Geometry check sheet. Reference: the model listing, model coordinates, mm. A direction names the side the tool comes from. Coordinates: 2 decimals unless noted, no trailing zeros. Write each loop counter-clockwise with the first axis right and the second up, starting at its lowest first coordinate (ties: lowest second). Pieces come first, ordered by that corner, then holes. Notation, with made-up numbers: (-9, -2) -> (-4, -2) arc R22 ccw to (-4, 7) -> close; hole circle Ø3 at (1, 53). An arc over 180 degrees is marked (long way). Use a Markdown table: item, result.
Autodesk Inventor part; units mm, degrees
ref_plane "Pracovní rovina2" through (15, 0, 0) normal (1, 0, 0) x (0, 0, -1)
ref_plane "YZ Plane" through (0, 0, 0) normal (1, 0, 0) x (0, 1, 0)
ref_plane "XZ Plane" through (0, 0, 0) normal (0, 1, 0) x (-1, 0, 0)
sketch "Náčrt1" plane through (0, 0, 0) normal (1, 0, 0) x (0, 1, 0)
  line L0 (0, 0) -> (100, 0)
  line L1 (100, 0) -> (100, -6)
  line L2 (100, -6) -> (6, -6)
  line L3 (6, -6) -> (6, -100)
  line L4 (6, -100) -> (0, -100)
  line L5 (0, -100) -> (0, 0)
  point P0 (100, -148)
  point P1 (100, -150)
  dimension "d0" = 100
  dimension "d1" = 6
  dimension "d20" = 100
  dimension "d40" = 6
  dimension "d108" = 94
  dimension "d109" = 94
extrude "Vysunutí1" add sketch "Náčrt1" along normal blind 140
sketch "Náčrt7" plane through (0, 6, -6) normal (0, 0, -1) x (-1, 0, 0)
  circle A0 centre (-125, 23) radius 5.25
  line L0 (0, 0) -> (-140, 0)
  line L1 (-140, 0) -> (-140, 94)
  line L2 (0, 94) -> (0, 0)
  point P0 (0, -6)
  dimension "d43" = 10.5
  dimension "d44" = 23
  dimension "d101" = 15
extrude "Vysunutí6" cut sketch "Náčrt7" against normal through all
sketch "Náčrt11" plane through (0, 0, 0) normal (-1, 0, 0) x (0, 0, 1)
  line L0 (0, 0) -> (0, 100)
  line L1 (0, 100) -> (-6, 100)
  line L2 (-6, 100) -> (-6, 6)
  line L3 (-6, 6) -> (-100, 6)
  line L4 (-100, 6) -> (-100, 0)
  line L5 (-100, 0) -> (0, 0)
extrude "Vysunutí9" add sketch "Náčrt11" along normal blind 110
sketch "Náčrt9" plane through (0, 6, -6) normal (0, 1, 0) x (1, 0, 0)
  line L0 (140, 94) -> (-110, 94)
  line L1 (140, -6) -> (140, 94)
  line L2 (-110, -6) -> (140, -6)
  line L3 (0, -6) -> (140, -6)
  arc A0 (5, 71.75) -> (5, 82.25) centre (5, 77) ccw
  arc A1 (-5, 82.25) -> (-5, 71.75) centre (-5, 77) ccw
  line L4 (-5, 71.75) -> (5, 71.75)
  line L5 (5, 82.25) -> (-5, 82.25)
  line L6 (-110, 94) -> (-110, -6)
  point P0 (0, -3)
  point P1 (0, 77)
  dimension "d89" = 140
  dimension "d91" = 10.5
  dimension "d92" = 10.5
  dimension "d93" = 10
  dimension "d94" = 5
  dimension "d106" = 17
sketch "Náčrt10" plane through (0, 0, 0) normal (0, 0, 1) x (1, 0, 0)
  line L0 (0, 100) -> (140, 100)
  circle A0 centre (125, 29) radius 5.25
  circle A1 centre (15, 75) radius 4.25
  arc A2 (-28.9496, 86.7763) -> (58.9496, 86.7763) centre (15, 75) ccw
  arc A3 (-38.6089, 89.3645) -> (68.6089, 89.3645) centre (15, 75) ccw
  arc A4 (68.6089, 89.3645) -> (58.9496, 86.7763) centre (63.7793, 88.0704) ccw
  line L1 (15, 75) -> (84.9162, 75)
  line L2 (15, 75) -> (59.3726, 86.8896)
  line L3 (15, 75) -> (15, -2.5844)
  line L4 (15, 75) -> (-28.9496, 86.7763)
  arc A5 (-28.9496, 86.7763) -> (-38.6089, 89.3645) centre (-33.7793, 88.0704) ccw
  line L5 (140, 100) -> (140, 0)
  line L6 (0, 0) -> (140, 0)
  dimension "d66" = 8.5
  dimension "d67" = 91
  dimension "d68" = 111
  dimension "d69" = 10
  dimension "d70" = 10
  dimension "d73" = 15
  dimension "d74" = 105
  dimension "d78" = 10
  dimension "d83" = 125
  dimension "d84" = 75
extrude "Vysunutí13" cut sketch "Náčrt9" against normal through all contours L4 A1 L5 A0
extrude "Vysunutí14" cut sketch "Náčrt10" against normal through all contours L1 L2 A1 | A1 L3 L1 | L2 L4 A1 | A1 L4 L3 | L1 A3 L3 A2 | A2 A4 A3 L1 | L3 A3 A5 A2
ref_plane "Pracovní rovina2" through (15, 0, 0) normal (1, 0, 0) x (0, 0, -1)
mirror "Zrcadlit2" about plane through (15, 0, 0) normal (1, 0, 0) of "Vysunutí13", "Vysunutí6"
sketch "Náčrt12" plane through (140, 6, -6) normal (0, 1, 0) x (1, 0, 0)
  line L0 (-115, 82.25) -> (-105, 82.25)
  arc A0 (-105, 71.75) -> (-105, 82.25) centre (-105, 77) ccw
  line L1 (-105, 71.75) -> (-115, 71.75)
  arc A1 (-115, 82.25) -> (-115, 71.75) centre (-115, 77) ccw
  line L2 (-135, 71.75) -> (-145, 71.75)
  arc A2 (-145, 82.25) -> (-145, 71.75) centre (-145, 77) ccw
  line L3 (-145, 82.25) -> (-135, 82.25)
  arc A3 (-135, 71.75) -> (-135, 82.25) centre (-135, 77) ccw
  line L4 (0, 0) -> (-250, 0)
  line L5 (0, 94) -> (0, 0)
  line L6 (0, 94) -> (-250, 94)
  line L7 (-250, 0) -> (-250, 94)
  circle A4 centre (-15, 77) radius 5.25
  point P0 (-140, -6)
  dimension "d102" = 10.5
  dimension "d103" = 15
  dimension "d107" = 17
extrude "Vysunutí15" cut sketch "Náčrt12" against normal through all contours A4
mirror "Zrcadlit3" about plane through (15, 0, 0) normal (1, 0, 0) of "Vysunutí15"
properties part number "L profil"
Item 1: Mould release check, pull along Y, two halves, no side actions. Record for faces 4 (the cylindrical face through (130, 3, -84.6)), 5 (the cylindrical face through (-32.38, 92.87, -2.96)), 6 (the cylindrical face through (13.58, 19.52, -2.96)), 7 (the flat face through (17, 6, -52)): +Y half, -Y half, draft (parallel to the pull), parting line (faces both ways), or undercut.
Answer block:
| item | result |
|---|---|
| face 4 | draft |
| face 5 | undercut |
| face 6 | undercut |
| face 7 | +Y half |
Item 2: Section check B-B on x = -95. Record the boundary of the cut face in (y, z).
Answer block:
| item | result |
|---|---|
| outline | (0, -100) -> (6, -100) -> (6, -88.25) -> (0, -88.25) -> close; (0, -77.75) -> (6, -77.75) -> (6, -6) -> (23.75, -6) -> (23.75, 0) -> (0, 0) -> close; (34.25, -6) -> (100, -6) -> (100, 0) -> (34.25, 0) -> close |
Item 3: Section check D-D on x = 84. Record the boundary of the cut face in (y, z).
Answer block:
| item | result |
|---|---|
| outline | (0, -100) -> (6, -100) -> (6, -6) -> (100, -6) -> (100, 0) -> (0, 0) -> close |
Item 4: Tool access check on faces 1 (the flat face through (17, 49, 0)), 2 (the flat face through (17, 54, -6)), 3 (the flat face through (30, 3, -77.75)). Record the directions out of +Z, -Z, +X, -X, +Y, -Y that give a thin tool (end or side, any length) a straight path to the whole face; none if there is none.
Answer block:
| item | result |
|---|---|
| face 1 | +Z, +X, -X, +Y, -Y |
| face 2 | -Z, +X, -X, +Y |
| face 3 | +Y, -Y |
Item 5: Depth check by flat-ended pin: P1, Ø5, axis at x = 107.5, z = -16, coming from the +Y side; P2, Ø7, axis at x = 15, y = 75, coming from the +Z side; P3, Ø12, axis at x = 125, z = -83, coming from the -Y side. Enter the tip coordinate at first touch or a pass-through.
Answer block:
| item | result |
|---|---|
| P1 | stops at y = 6 |
| P2 | passes through |
| P3 | stops at y = 0 |
Item 6: Thickness scan on L1, parallel to Y at x = 15, z = -1.25; L2, parallel to X at y = 3, z = -83; L3, parallel to Y at x = 125, z = -4. Record the ranges inside material, lowest first. Write a range as [from, to].
Answer block:
| item | result |
|---|---|
| L1 | y = [0, 19.5], [29.5, 70.75], [79.25, 100] |
| L2 | x = [-110, -100.25], [-89.75, -10.25], [10.25, 19.75], [40.25, 119.75], [130.25, 140] |
| L3 | y = [0, 23.75], [34.25, 100] |
Item 7: Section check A-A on z = -83. Record the boundary of the cut face in (x, y).
Answer block:
| item | result |
|---|---|
| outline | (-110, 0) -> (-100.25, 0) -> (-100.25, 6) -> (-110, 6) -> close; (-89.75, 0) -> (-10.25, 0) -> (-10.25, 6) -> (-89.75, 6) -> close; (10.25, 0) -> (19.75, 0) -> (19.75, 6) -> (10.25, 6) -> close; (40.25, 0) -> (119.75, 0) -> (119.75, 6) -> (40.25, 6) -> close; (130.25, 0) -> (140, 0) -> (140, 6) -> (130.25, 6) -> close |
Item 8: Section check C-C on x = -17. Record the boundary of the cut face in (y, z).
Answer block:
| item | result |
|---|---|
| outline | (0, -100) -> (6, -100) -> (6, -6) -> (29.65, -6) -> (29.65, 0) -> (0, 0) -> close; (42.65, -6) -> (100, -6) -> (100, 0) -> (42.65, 0) -> close |
